The listing builds one solid part. Answer for the finished solid, in the listing's coordinates (mm). A direction names the side the tool comes from. Give positions to 0.01 mm unless a question says otherwise; leave off trailing zeros. Write each loop counter-clockwise with the first axis right and the second up, starting at its lowest first coordinate (ties: lowest second). Pieces come first, ordered by that corner, then holes. Notation, with made-up numbers: M 58,78.5 L 94,78.5 A21 cw 94,115.5 Z; hole C -18,-33.75 d4. An arc over 180 degrees is marked long. Return JSON: item names as keys, results as strings.
from build123d import *

# Parameters (mm, degrees)
BOSS_EXTRUDE1_DEPTH = 11.5
SKETCH1_13_R        = 1.5
SKETCH1_13_R_2      = 1.25
BOSS_EXTRUDE2_DEPTH = 7.75
BOSS_EXTRUDE3_DEPTH = 7
SKETCH2_R           = 1.5
BOSS_EXTRUDE4_DEPTH = 5


with BuildPart() as part:
    # Sketch1 → Boss-Extrude1 (new body, symmetric)
    with BuildSketch(Plane(origin=(0, 0, 0), x_dir=(1, 0, 0), z_dir=(0, 1, 0))):
        with BuildLine():
            Line((6.824314586, 7.284360201), (6.824314586, 9.00020274))
            Line((6.824314586, 9.00020274), (-3.690467309, 9.00020274))
            Line((-3.690467309, 9.00020274), (-17.038497557, 11.5))
            Line((-17.038497557, 11.5), (-24.867971487, 11.5))
            Line((-24.867971487, 11.5), (-24.867971487, -11.5))
            Line((-24.867971487, -11.5), (-17.038497557, -11.5))
            Line((-17.038497557, -11.5), (-3.690467309, -9.00020274))
            Line((-3.690467309, -9.00020274), (6.824314586, -9.00020274))
            Line((6.824314586, -9.00020274), (6.824314586, -7.284360201))
            ThreePointArc((6.824314586, -7.284360201), (4.861171432, -6.879883717), (3.082035449, -5.956732906))
            Line((3.082035449, -5.956732906), (-3.422402494, -3.4))
            Line((-3.422402494, -3.4), (-19.513448301, -3.4))
            Line((-19.513448301, -3.4), (-19.513448301, 3.4))
            Line((-19.513448301, 3.4), (-3.422402494, 3.4))
            Line((-3.422402494, 3.4), (3.082035449, 5.956732906))
            ThreePointArc((3.082035449, 5.956732906), (4.861171432, 6.879883717), (6.824314586, 7.284360201))
        make_face()
    extrude(amount=BOSS_EXTRUDE1_DEPTH, both=True)

    # Sketch1_13 → Boss-Extrude2 (add, symmetric)
    with BuildSketch(Plane(origin=(0, 0, 0), x_dir=(1, 0, 0), z_dir=(0, 1, 0))):
        with BuildLine():
            Line((6.824314586, 3.971385595), (6.824314586, 7.284360201))
            ThreePointArc((6.824314586, 7.284360201), (4.861171432, 6.879883717), (3.082035449, 5.956732906))
            Line((3.082035449, 5.956732906), (-3.422402494, 3.4))
            Line((-3.422402494, 3.4), (-19.513448301, 3.4))
            Line((-19.513448301, 3.4), (-19.513448301, -3.4))
            Line((-19.513448301, -3.4), (-3.422402494, -3.4))
            Line((-3.422402494, -3.4), (3.082035449, -5.956732906))
            ThreePointArc((3.082035449, -5.956732906), (4.861171432, -6.879883717), (6.824314586, -7.284360201))
            Line((6.824314586, -7.284360201), (6.824314586, -3.971385595))
            ThreePointArc((6.824314586, -3.971385595), (3.301909035, 0), (6.824314586, 3.971385595))
        make_face()
        with Locations((-17.038497557, 0)):
            Circle(SKETCH1_13_R, mode=Mode.SUBTRACT)
        with Locations((-13.038497557, 0)):
            Circle(SKETCH1_13_R, mode=Mode.SUBTRACT)
        with Locations((-2.172402494, 0)):
            Circle(SKETCH1_13_R_2, mode=Mode.SUBTRACT)
    extrude(amount=BOSS_EXTRUDE2_DEPTH, both=True)

    # Sketch1_14 → Boss-Extrude3 (add, symmetric)
    with BuildSketch(Plane(origin=(0, 0, 0), x_dir=(1, 0, 0), z_dir=(0, 1, 0))):
        with BuildLine():
            Line((6.824314586, -3.971385595), (6.824314586, 3.971385595))
            ThreePointArc((6.824314586, 3.971385595), (3.301909035, 0), (6.824314586, -3.971385595))
        make_face()
    extrude(amount=BOSS_EXTRUDE3_DEPTH, both=True)

    # Sketch2 → Boss-Extrude4 (add)
    with BuildSketch(Plane.ZY.offset(24.867971487)):
        Polygon((0.8, 5.69251999), (-10.999928788, 5.69251999), (-10.999928788, -5.69251999), (0.8, -5.69251999), (0.8, -5.7), (5.6, -5.7), (5.6, -8.6), (11, -8.6), (11, 8.6), (5.6, 8.6), (5.6, 5.7), (0.8, 5.7), align=None)
        with Locations((-5.3, 0)):
            Circle(SKETCH2_R, mode=Mode.SUBTRACT)
    extrude(amount=BOSS_EXTRUDE4_DEPTH)


solid = part.part
Item 1: Determine the mould class of faces 1 (the cylindrical face through (-18.537, -0.109, -0.066)), 2 (the flat face through (-0.12, -9.6, 4.7)), 3 (the flat face through (-12, -10, -3.4)) for opening direction X: +X half, -X half, draft (parallel to the pull), parting line (faces both ways), or undercut.
Geometry results:
{"face 1": "undercut", "face 2": "+X half", "face 3": "draft"}
Item 2: Find the intervals of material crossed by line 1 (X direction, y = -3.75, z = 0); line 2 (X direction, y = 5, z = -0.5); line 3 (Z direction, x = 3.5, y = -10.25), in increasing order.
Geometry results:
{"line 1": "x = -29.87 to -18.54, -15.54 to -14.54, -11.54 to -3.42, -0.92 to 6.82", "line 2": "x = -29.87 to -18.45, -15.62 to -14.45, -11.62 to -3.32, -1.03 to 6.82", "line 3": "z = -9 to -6.23, 6.23 to 9"}
Item 3: A cutting plane is placed at C-C, the plane y = -9.75. Write down the section's boundary in (x, z), plus the area to 3 significant figures.
Geometry results:
{"outline": "M -24.87,-11.5 L -17.04,-11.5 L -3.69,-9 L 6.82,-9 L 6.82,-7.28 A7.3 cw 3.08,-5.96 L -3.42,-3.4 L -19.51,-3.4 L -19.51,3.4 L -3.42,3.4 L 3.08,5.96 A7.3 cw 6.82,7.28 L 6.82,9 L -3.69,9 L -17.04,11.5 L -24.87,11.5 Z", "area": "422 mm2"}
Item 4: A cutting plane is placed at A-A, the plane y = 0. Write down the section's boundary in (x, z), plus the area to 3 significant figures.
Geometry results:
{"outline": "M -29.87,-11 L -24.87,-11 L -24.87,-11.5 L -17.04,-11.5 L -3.69,-9 L 6.82,-9 L 6.82,9 L -3.69,9 L -17.04,11.5 L -24.87,11.5 L -24.87,11 L -29.87,11 L -29.87,-3.8 L -24.87,-3.8 L -24.87,-6.8 L -29.87,-6.8 Z; hole C -17.04,0 d3; hole C -13.04,0 d3; hole C -2.17,0 d2.5", "area": "719 mm2"}
Item 5: A cutting plane is placed at D-D, the plane x = -17.5. Write down the section's boundary in (y, z).
Geometry results:
{"outline": "M -11.5,-11.5 L 11.5,-11.5 L 11.5,-3.4 L 7.75,-3.4 L 7.75,-1.43 L -7.75,-1.43 L -7.75,-3.4 L -11.5,-3.4 Z; M -11.5,3.4 L -7.75,3.4 L -7.75,1.43 L 7.75,1.43 L 7.75,3.4 L 11.5,3.4 L 11.5,11.5 L -11.5,11.5 Z"}
Item 6: A cutting plane is placed at B-B, the plane z = 0. Write down the section's boundary in (x, y), plus the area to 3 significant figures.
Geometry results:
{"outline": "M -29.87,-5.69 L -24.87,-5.69 L -24.87,-11.5 L -19.51,-11.5 L -19.51,-7.75 L -18.54,-7.75 L -18.54,7.75 L -19.51,7.75 L -19.51,11.5 L -24.87,11.5 L -24.87,5.69 L -29.87,5.69 Z; M -15.54,-7.75 L -14.54,-7.75 L -14.54,7.75 L -15.54,7.75 Z; M -11.54,-7.75 L -3.42,-7.75 L -3.42,7.75 L -11.54,7.75 Z; M -0.92,-7.75 L 3.3,-7.75 L 3.3,-7 L 6.82,-7 L 6.82,7 L 3.3,7 L 3.3,7.75 L -0.92,7.75 Z", "area": "451 mm2"}
Item 7: Given pin 1 Ø1.1 at (y, z) = (-9, -0.5) entering from +X; pin 2 Ø1.1 at (x, y) = (-13.5, 9) entering from +Z; pin 3 Ø4 at (x, y) = (-12, 9) entering from -Z, each flat-ended and moving along its own axis, determine where each tip first touches the part or whether it passes through.
Geometry results:
{"pin 1": "stops at x = -19.51", "pin 2": "stops at z = 10.94", "pin 3": "stops at z = -10.93"}
Item 8: Which of the six approach directions +Z, -Z, +X, -X, +Y, -Y give full straight-line access (tool end or side, diameter ignored) to faces 4 (the flat face through (2, 0, -9)), 5 (the flat face through (-27, -8.6, 8)), 6 (the flat face through (-0.22, -9.6, -4.66))?
Geometry results:
{"face 4": "-Z, +X, +Y, -Y", "face 5": "+Z, -Z, -X, -Y", "face 6": "+X, -Y"}
